For this review, take the finished solid that the model builds, in its own axes (mm). Face numbers are marked on the shaded views. A direction names the side the tool comes from. Give positions to 0.01 mm unless a question says otherwise; leave off trailing zeros. Order: outer loops, then holes, each group sorted by start corner. A loop starts at its lowest first (then second) coordinate and runs counter-clockwise, first axis right, second up.
from build123d import *

# Parameters (mm, degrees)
F0_R     = 102.5
F1_DEPTH = 25
F2_DEPTH = 1
F3_DEPTH = 25
F4_R     = 102.5
F4_R_2   = 97.5
F5_DEPTH = 10


with BuildPart() as f1:
    # F0 (on Top) → F1 (new body)
    with BuildSketch(Plane.XY):
        with BuildLine():
            Line((160, 160), (2.52e-08, 160))
            ThreePointArc((2.52e-08, 160), (113.1370849988, 113.1370849809), (160, 0))
            Line((160, 0), (160, 160))
        make_face()
        with BuildLine():
            ThreePointArc((160, 0), (113.1370849988, 113.1370849809), (2.52e-08, 160))
            ThreePointArc((2.52e-08, 160), (-113.13708472, 113.1370852597), (-160, 7.381e-07))
            ThreePointArc((-160, 7.381e-07), (-113.1370852131, -113.1370847666), (1.067e-07, -160))
            ThreePointArc((1.067e-07, -160), (113.1370850276, -113.1370849521), (160, 0))
        make_face()
        Circle(F0_R, mode=Mode.SUBTRACT)
        with BuildLine():
            Line((160, -160), (160, 0))
            ThreePointArc((160, 0), (113.1370850276, -113.1370849521), (1.067e-07, -160))
            Line((1.067e-07, -160), (160, -160))
        make_face()
        Circle(F0_R)
        with BuildLine():
            Line((2.52e-08, 160), (-160, 160))
            Line((-160, 160), (-160, 7.381e-07))
            ThreePointArc((-160, 7.381e-07), (-113.13708472, 113.1370852597), (2.52e-08, 160))
        make_face()
        with BuildLine():
            ThreePointArc((1.067e-07, -160), (-113.1370852131, -113.1370847666), (-160, 7.381e-07))
            Line((-160, 7.381e-07), (-160, -160))
            Line((-160, -160), (1.067e-07, -160))
        make_face()
    extrude(amount=-F1_DEPTH)

    # F0 (on Top) → F2 (join)
    with BuildSketch(Plane.XY):
        with BuildLine():
            ThreePointArc((160, 0), (113.1370849988, 113.1370849809), (2.52e-08, 160))
            ThreePointArc((2.52e-08, 160), (-113.13708472, 113.1370852597), (-160, 7.381e-07))
            ThreePointArc((-160, 7.381e-07), (-113.1370852131, -113.1370847666), (1.067e-07, -160))
            ThreePointArc((1.067e-07, -160), (113.1370850276, -113.1370849521), (160, 0))
        make_face()
        Circle(F0_R, mode=Mode.SUBTRACT)
    extrude(amount=F2_DEPTH)

    # F3 (cut): a face of the model
    f3_faces = [f1.faces().sort_by_distance(p)[0] for p in [
        (0, 0, 0),
    ]]
    extrude(f3_faces, amount=-F3_DEPTH, mode=Mode.SUBTRACT)

    # F4 (on Top) → F5 (join)
    with BuildSketch(Plane.XY):
        Circle(F4_R)
        Circle(F4_R_2, mode=Mode.SUBTRACT)
    extrude(amount=-F5_DEPTH)


solid = f1.part
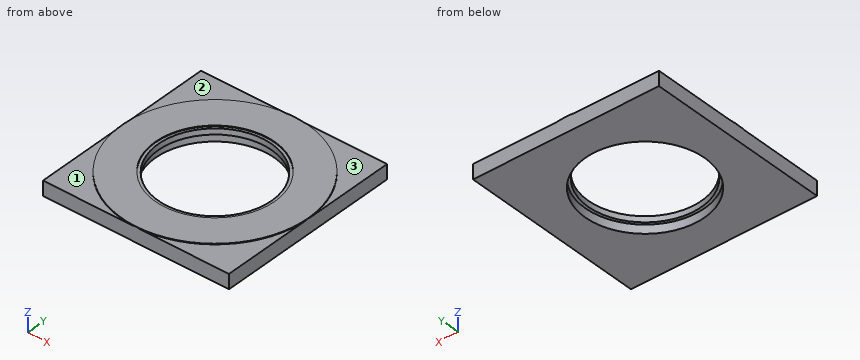
1) We need section C-C on z = -18.5. Give the boundary of the cut face in (x, y), then the cut area to 3 significant figures.
Answer sheet:
outline: (-160, -160) - (160, -160) - (160, 160) - (-160, 160) - close; hole circle Ø205 at (0, 0)
area: 69,400 mm2
2) We need section B-B on x = 70.5. Give the boundary of the cut face in (y, z), then the cut area to 3 significant figures.
Answer sheet:
outline: (-160, -25) - (-74.4, -25) - (-74.4, -10) - (-67.35, -10) - (-67.35, 0) - (-74.4, 0) - (-74.4, 1) - (-143.63, 1) - (-143.63, 0) - (-160, 0) - close; (67.35, -10) - (74.4, -10) - (74.4, -25) - (160, -25) - (160, 0) - (143.63, 0) - (143.63, 1) - (74.4, 1) - (74.4, 0) - (67.35, 0) - close
area: 4,560 mm2
3) Tool access review of the marked faces 1, 2 and 3: name each direction out of +Z, -Z, +X, -X, +Y, -Y from which nothing blocks a thin tool from reaching the whole face with its end or side.
Answer sheet:
face 1: +Z, -X, -Y
face 2: +Z, -X, +Y
face 3: +Z, +X, +Y
4) We need section A-A on y = -64.5. Give the boundary of the cut face in (x, z).
Answer sheet:
outline: (-160, -25) - (-79.66, -25) - (-79.66, -10) - (-73.12, -10) - (-73.12, 0) - (-79.66, 0) - (-79.66, 1) - (-146.42, 1) - (-146.42, 0) - (-160, 0) - close; (73.12, -10) - (79.66, -10) - (79.66, -25) - (160, -25) - (160, 0) - (146.42, 0) - (146.42, 1) - (79.66, 1) - (79.66, 0) - (73.12, 0) - close
5) To check wall thickness, follow line 1 (Y direction, x = 0, z = -17.75); line 2 (Y direction, x = 0, z = -1.75); line 3 (X direction, y = -60.5, z = -15). State the ranges of each line that lie inside material, in increasing order.
Answer sheet:
line 1: y = -160 to -102.5, 102.5 to 160
line 2: y = -160 to -97.5, 97.5 to 160
line 3: x = -160 to -82.74, 82.74 to 160
6) We need section D-D on y = -133.5. Give the boundary of the cut face in (x, z).
Answer sheet:
outline: (-160, -25) - (160, -25) - (160, 0) - (88.19, 0) - (88.19, 1) - (-88.19, 1) - (-88.19, 0) - (-160, 0) - close
